from build123d import *

# Parameters (mm, degrees)
BASPROSKE_W             = 10
BASPROSKE_H             = 11
TOOTHCUT_DEPTH          = 19.493242009
TEETHCUTS_COUNT         = 20
TEETHCUTS_ANGLE         = 342
BORSKE_R                = 0.4
BORE_DEPTH              = 50.0000508
SKETCH1_R               = 6.25
BOSS_EXTRUDE1_DEPTH     = 5
CUT_EXTRUDE1_DEPTH      = 19.376827944
CUT_EXTRUDE1_DEPTH_BACK = 19.376827944
FILLET1_R               = 0.5
CHAMFER1_SIZE           = 0.5
FILLET2_R               = 0.25


with BuildPart() as part:
    # BasProSke → Base-Revolve (revolve)
    with BuildSketch(Plane(origin=(0, 0, 0), x_dir=(1, 0, 0), z_dir=(0, 1, 0)), mode=Mode.PRIVATE) as base_revolve_sk:
        with Locations((5, 5.5)):
            Rectangle(BASPROSKE_W, BASPROSKE_H)
    revolve(base_revolve_sk.sketch.rotate(Axis((-10, 0, 0), (1, 0, 0)), 180), axis=Axis((-10, 0, 0), (1, 0, 0)))

    # TooCutSke → ToothCut (cut, through all)
    with BuildSketch(Plane(origin=(0, 0, 0), x_dir=(0, 0, -1), z_dir=(1, 0, 0))):
        with BuildLine():
            ThreePointArc((0.499924007, 8.734705318), (0, 8.749), (-0.499924007, 8.734705318))
            ThreePointArc((-0.499924007, 8.734705318), (-0.824302243, 9.905497836), (-1.485192705, 10.924909509))
            ThreePointArc((-1.485192705, 10.924909509), (0, 11.0254), (1.485192705, 10.924909509))
            ThreePointArc((1.485192705, 10.924909509), (0.824302243, 9.905497836), (0.499924007, 8.734705318))
        make_face()
    toothcut = extrude(amount=TOOTHCUT_DEPTH, mode=Mode.SUBTRACT)

    # TeethCuts: ToothCut ×20 about axis
    teethcuts_axis = Axis((-10, 0, 0), (1, 0, 0))
    for i in range(1, TEETHCUTS_COUNT):
        add(toothcut.rotate(teethcuts_axis, i * TEETHCUTS_ANGLE / (TEETHCUTS_COUNT - 1)), mode=Mode.SUBTRACT)

    # BorSke → Bore (cut, symmetric)
    with BuildSketch(Plane(origin=(0, 0, 0), x_dir=(0, 0, -1), z_dir=(1, 0, 0))):
        with Locations(Location((0, 0, 0), (0, 0, 180))):
            Circle(BORSKE_R)
    extrude(amount=BORE_DEPTH, both=True, mode=Mode.SUBTRACT)

    # Sketch1 → Boss-Extrude1 (add)
    with BuildSketch(Plane.ZY):
        with Locations(Location((0, 0, 0), (0, 0, 180))):
            Circle(SKETCH1_R)
    extrude(amount=BOSS_EXTRUDE1_DEPTH)

    # Sketch2 → Cut-Extrude1 (cut, two sides)
    with BuildSketch(Plane(origin=(0, 0, 0), x_dir=(0, 0, -1), z_dir=(1, 0, 0))) as cut_extrude1_sk:
        Polygon((-2.5, -1.443375673), (2.5, -1.443375673), (0, 2.886751346), align=None)
    extrude(amount=CUT_EXTRUDE1_DEPTH, mode=Mode.SUBTRACT)
    extrude(cut_extrude1_sk.sketch, amount=-CUT_EXTRUDE1_DEPTH_BACK, mode=Mode.SUBTRACT)

    # Fillet1
    fillet1_edges = [part.edges().sort_by_distance(p)[0] for p in [
        (0, 0, 6.25),
    ]]
    fillet(fillet1_edges, radius=FILLET1_R)

    # Chamfer1
    chamfer1_edges = [part.edges().sort_by_distance(p)[0] for p in [
        (-5, 0, 6.25),
    ]]
    chamfer(chamfer1_edges, length=CHAMFER1_SIZE)

    # Fillet2
    fillet2_edges = [part.edges().sort_by_distance(p)[0] for p in [
        (2.5, -1.443375673, 2.5),
        (2.5, 2.886751346, 0),
        (2.5, -1.443375673, -2.5),
    ]]
    fillet(fillet2_edges, radius=FILLET2_R)


solid = part.part
The model under review builds one solid part; all positions refer to its coordinate system, in mm. A direction names the side the tool comes from. Coordinates: 2 decimals unless noted, no trailing zeros. Loops run counter-clockwise (first coordinate to the right, second up) from the corner with the lowest first, then second, coordinate; pieces in that order, holes last.
(1) Draft analysis for pull direction Z (two halves, no side actions). For faces 1 (the cylindrical face through (4.93, -2.28, -9.64)), 2 (the cylindrical face through (4.93, 6.49, 7.53)), 3 (the cylindrical face through (4.93, -3.85, -9.17)), 4 (the cylindrical face through (4.93, 7.53, -6.49)), state which applies: +Z half, -Z half, draft (parallel to the pull), parting line (faces both ways), or undercut.
Determined:
face 1: undercut
face 2: +Z half
face 3: -Z half
face 4: undercut
(2) Consider section B-B, the plane y = 0. Give the boundary of the cut face in (x, z).
Determined:
outline: (-5, -5.75) - (-4.5, -6.25) - (-0.5, -6.25) arc R0.5 cw to (0, -6.75) - (0, -8.75) - (10, -8.75) - (10, -1.67) - (-5, -1.67) - close; (-5, 1.67) - (10, 1.67) - (10, 8.75) - (0, 8.75) - (0, 6.75) arc R0.5 cw to (-0.5, 6.25) - (-4.5, 6.25) - (-5, 5.75) - close
(3) Insertion check: P1, Ø5, axis at x = 4, y = -5, coming from the -Z side; P2, Ø4, axis at x = 0.5, z = -6, coming from the -Y side; P3, Ø4, axis at x = 4, y = -7.5, coming from the -Z side. Each pin has a flat end and moves straight along its axis. Give the tip position at first contact, or say it passes through.
Determined:
P1: stops at z = -9.92
P2: stops at y = -9.92
P3: stops at z = -7.96
(4) Consider section A-A, the plane x = -2.5. Give the boundary of the cut face in (y, z), plus the area to 3 significant figures.
Determined:
outline: circle Ø12.5 at (0, 0); hole (-1.44, -2.07) arc R0.25 ccw to (-1.07, -2.28) - (2.51, -0.22) arc R0.25 ccw to (2.51, 0.22) - (-1.07, 2.28) arc R0.25 ccw to (-1.44, 2.07) - close
area: 112 mm2
(5) Wall thickness on L1, parallel to Z at x = 2.5, y = -7; L2, parallel to Y at x = 1.5, z = -7.5; L3, parallel to X at y = 8.25, z = 5: over which ranges is each line inside the solid? List them lowest first.
Determined:
L1: z = -7.78 to -5.77, -5.25 to 5.25, 5.77 to 7.78
L2: y = -7.94 to -6.44, -4.8 to 4.8, 6.44 to 7.94
L3: x = 0 to 10
(6) Tool access review of faces 5 (the cylindrical face through (4.93, -3.82, 9.14)), 6 (the flat face through (0, 7, 0)), 7 (the cylindrical face through (4.93, -9.64, 2.28)), 8 (the cylindrical face through (4.93, -9.14, -3.82)): name each direction out of +Z, -Z, +X, -X, +Y, -Y from which nothing blocks a thin tool from reaching the whole face with its end or side.
Determined:
face 5: +Z, +X, -X
face 6: -X
face 7: +X, -X
face 8: +X, -X, -Y
